Source: CAD feature listing. Evaluate the final solid. Frame: model axes, mm. A direction names the side the tool comes from. Coordinates: 2 decimals unless noted, no trailing zeros. Loops run counter-clockwise (first coordinate to the right, second up) from the corner with the lowest first, then second, coordinate; pieces in that order, holes last. Notation, with made-up numbers: M 39.25,58 L 84.25,58 A20 ccw 84.25,89 Z; hole C 67,79 d5. An arc over 180 degrees is marked long. Write each question's results on one line, items separated by ' | '. Start each with the question number.
from build123d import *

# Parameters (mm, degrees)
DODANIE_WYCI_GNI_CIE1_DEPTH = 0.4
WYTNIJ_WYCI_GNI_CIE1_REACH  = 11.06
SZKIC6_R                    = 4
DODANIE_WYCI_GNI_CIE4_DEPTH = 0.4


with BuildPart() as part:
    # Szkic1 → Dodanie-wyciągnięcie1 (new body)
    with BuildSketch(Plane.XY):
        with BuildLine():
            Line((0, -6.4), (6.4, -6.4))
            Line((6.4, -6.4), (6.4, 0))
            ThreePointArc((6.4, 0), (0, 6.4), (-6.4, 0))
            Line((-6.4, 0), (-6.4, -6.4))
            Line((-6.4, -6.4), (0, -6.4))
        make_face()
    extrude(amount=DODANIE_WYCI_GNI_CIE1_DEPTH)

    # Szkic6 → Wytnij-wyciągnięcie1 (cut, up to next)
    with BuildSketch(Plane.XY.offset(0.4), mode=Mode.PRIVATE) as wytnij_wyci_gni_cie1_sk1:
        Circle(SZKIC6_R)
    wytnij_wyci_gni_cie1_tool1 = extrude(wytnij_wyci_gni_cie1_sk1.sketch, amount=-WYTNIJ_WYCI_GNI_CIE1_REACH, mode=Mode.PRIVATE) & part.part
    add(wytnij_wyci_gni_cie1_tool1.solids().sort_by_distance((0, 0, 0.4))[0], mode=Mode.SUBTRACT)

    # Szkic5 → Dodanie-wyciągnięcie4 (add)
    with BuildSketch(Plane.ZY.offset(6.4)):
        with BuildLine():
            Line((5.000724361, -6.56862155), (5.000724361, -8))
            ThreePointArc((5.000724361, -8), (4.956790379, -8.106066017), (4.850724361, -8.15))
            Line((4.850724361, -8.15), (4.600724361, -8.15))
            Line((4.600724361, -8.15), (5.112747467, -9.097540152))
            ThreePointArc((5.112747467, -9.097540152), (5.149509203, -9.135889508), (5.200724361, -9.15))
            Line((5.200724361, -9.15), (5.400724361, -9.15))
            ThreePointArc((5.400724361, -9.15), (5.468361913, -9.123655697), (5.500362181, -9.058503233))
            Line((5.500362181, -9.058503233), (5.850362181, -4.957329291))
            ThreePointArc((5.850362181, -4.957329291), (6.350362181, -4.498182514), (6.850362181, -4.957329291))
            Line((6.850362181, -4.957329291), (7.200362181, -9.058503233))
            ThreePointArc((7.200362181, -9.058503233), (7.232362449, -9.123655697), (7.3, -9.15))
            Line((7.3, -9.15), (7.5, -9.15))
            ThreePointArc((7.5, -9.15), (7.551215158, -9.135889508), (7.587976894, -9.097540152))
            Line((7.587976894, -9.097540152), (8.1, -8.15))
            Line((8.1, -8.15), (7.85, -8.15))
            ThreePointArc((7.85, -8.15), (7.743933983, -8.106066017), (7.7, -8))
            Line((7.7, -8), (7.7, -6.55))
            ThreePointArc((7.7, -6.55), (7.712395552, -6.464655511), (7.748557878, -6.386363636))
            Line((7.748557878, -6.386363636), (7.951442122, -6.074613587))
            ThreePointArc((7.951442122, -6.074613587), (7.987604448, -5.996321712), (8, -5.910977223))
            Line((8, -5.910977223), (8, 0.6))
            Line((8, 0.6), (6, 2.6))
            Line((6, 2.6), (0, 2.6))
            Line((0, 2.6), (0, -6.4))
            Line((0, -6.4), (3.450724361, -6.4))
            ThreePointArc((3.450724361, -6.4), (3.945699108, -6.194974747), (4.150724361, -5.7))
            Line((4.150724361, -5.7), (4.150724361, -5))
            ThreePointArc((4.150724361, -5), (4.400724361, -4.75), (4.650724361, -5))
            Line((4.650724361, -5), (4.650724361, -5.98137845))
            ThreePointArc((4.650724361, -5.98137845), (4.661549722, -6.046285735), (4.692853918, -6.104166573))
            Line((4.692853918, -6.104166573), (4.958594805, -6.445833427))
            ThreePointArc((4.958594805, -6.445833427), (4.989899001, -6.503714265), (5.000724361, -6.56862155))
        make_face()
    dodanie_wyci_gni_cie4 = extrude(amount=-DODANIE_WYCI_GNI_CIE4_DEPTH)

    # Lustro1: Dodanie-wyciągnięcie4 across plane
    add(dodanie_wyci_gni_cie4.mirror(Plane(origin=(0, 0, 0), x_dir=(0, 0, 1), z_dir=(1, 0, 0))))


solid = part.part
Item 1: First-contact query: pin 1 Ø2 at (x, z) = (-3.5, 2.5) entering from +Y; pin 2 Ø6 at (x, y) = (0.5, -1.5) entering from +Z. Flat tips, straight axial feed; report the tip coordinate or a pass-through.
Item 2: Cut plane A-A (x = 0). Output: boundary loops of the cut face in (y, z).
Item 3: Cut plane B-B (y = 0). Output: boundary loops of the cut face in (x, z).
Item 4: Cut plane C-C (z = 2.25). Output: boundary loops of the cut face in (x, y), then the cut area to 3 significant figures.
Item 5: Line query: probe 1 along X at (y, z) = (0.25, 5.5); probe 2 along Z at (x, y) = (-0.25, -6). Output: solid intervals per line, ascending.
Item 6: Mould query, pull axis X, two halves, no side actions, for faces 4 (the cylindrical face through (-0.867, -3.905, 0.203)), 5 (the flat face through (-6, -2, 4)), 6 (the flat face through (6.4, -2, 4)), 7 (the flat face through (-6.4, -2, 4)). Classes: +X half, -X half, draft (parallel to the pull), parting line (faces both ways), or undercut.
Item 7: Access query for faces 1 (the flat face through (-0.1, -4.2, 0.4)), 2 (the flat face through (0, -6.4, 0.2)), 3 (the flat face through (-6.2, 1.6, 7)). Directions: +Z, -Z, +X, -X, +Y, -Y. A direction counts if a zero-diameter tool reaches every point of the face in a straight line with its end or side. Return the directions, or none.
Item 8: Cut plane D-D (y = -5.5). Output: boundary loops of the cut face in (x, z), then the cut area to 3 significant figures.
Response values:
1) pin 1: passes through | pin 2: stops at z = 0.4
2) outline: M -6.4,0 L -4,0 L -4,0.4 L -6.4,0.4 Z; M 4,0 L 6.4,0 L 6.4,0.4 L 4,0.4 Z
3) outline: M -6.4,0 L -4,0 L -4,0.4 L -6,0.4 L -6,8 L -6.4,8 Z; M 4,0 L 6.4,0 L 6.4,8 L 6,8 L 6,0.4 L 4,0.4 Z
4) outline: M -6.4,-6.4 L -6,-6.4 L -6,2.6 L -6.4,2.6 Z; M 6,-6.4 L 6.4,-6.4 L 6.4,2.6 L 6,2.6 Z | area: 7.20 mm2
5) probe 1: x = -6.4 to -6, 6 to 6.4 | probe 2: z = 0 to 0.4
6) face 4: undercut | face 5: undercut | face 6: +X half | face 7: -X half
7) face 1: +Z, +Y, -Y | face 2: -Z, +X, -X, -Y | face 3: +Z, +X, -X, +Y
8) outline: M -6.4,0 L 6.4,0 L 6.4,4.15 L 6,4.15 L 6,0.4 L -6,0.4 L -6,4.15 L -6.4,4.15 Z; M -6.4,4.65 L -6,4.65 L -6,5.8 L -6.4,5.8 Z; M -6.4,6.9 L -6,6.9 L -6,8 L -6.4,8 Z; M 6,4.65 L 6.4,4.65 L 6.4,5.8 L 6,5.8 Z; M 6,6.9 L 6.4,6.9 L 6.4,8 L 6,8 Z | area: 9.93 mm2
